The listing builds one solid part. Answer for the finished solid, in the listing's coordinates (mm). Face numbers are marked on the shaded views. A direction names the side the tool comes from. Give positions to 0.01 mm unless a question says otherwise; leave off trailing zeros. Write each loop counter-clockwise with the first axis right and the second up, starting at its lowest first coordinate (ties: lowest second). Pieces come first, ordered by that corner, then holes. Notation, with made-up numbers: (30.5, 51.25) -> (74.5, 51.25) arc R17 cw to (74.5, 81.25) -> close; hole circle Ø11 at (-5, 7). An arc over 180 degrees is marked (long way). Use CSV: the item, a comma, the result in double quotes. Start each with the question number.
from build123d import *

# Parameters (mm, degrees)
CLAMP_EXTRUDE_DEPTH     = 10
HOLE_R                  = 1.6
HOLES_CUT_EXTRUDE_DEPTH = 6
FILLET1_R               = 1


with BuildPart() as part:
    # Sketch4 → Clamp Extrude (new body)
    with BuildSketch(Plane(origin=(0, 0, 0), x_dir=(0, 0, -1), z_dir=(1, 0, 0))):
        with BuildLine():
            Line((-23.6125, 0), (-11.1125, 0))
            ThreePointArc((-11.1125, 0), (0, -11.1125), (11.1125, 0))
            Line((11.1125, 0), (23.6125, 0))
            Line((23.6125, 0), (23.6125, -5))
            Line((23.6125, -5), (13.789947652, -5))
            ThreePointArc((13.789947652, -5), (0, -14.668423782), (-13.789947652, -5))
            Line((-13.789947652, -5), (-23.6125, -5))
            Line((-23.6125, -5), (-23.6125, 0))
        make_face()
    extrude(amount=CLAMP_EXTRUDE_DEPTH)

    # Hole → Holes Cut-Extrude (cut, through all)
    with BuildSketch(Plane.XZ.offset(5)):
        with Locations((5, 18.701223826)):
            Circle(HOLE_R)
        with Locations((5, -18.701223826)):
            Circle(HOLE_R)
    extrude(amount=-HOLES_CUT_EXTRUDE_DEPTH, mode=Mode.SUBTRACT)

    # Fillet1
    fillet1_edges = [part.edges().sort_by_distance(p)[0] for p in [
        (0, -2.5, -23.6125),
        (0, -5, -18.701223826),
        (0, -14.668423782, 0),
        (10, -2.5, -23.6125),
        (5, -5, 13.789947652),
        (5, -5, 23.6125),
        (5, -5, -23.6125),
        (5, -5, -13.789947652),
        (10, -2.5, 23.6125),
        (10, -5, 18.701223826),
        (10, -14.668423782, 0),
        (0, -5, 18.701223826),
        (10, -5, -18.701223826),
        (0, -2.5, 23.6125),
    ]]
    fillet(fillet1_edges, radius=FILLET1_R)


solid = part.part
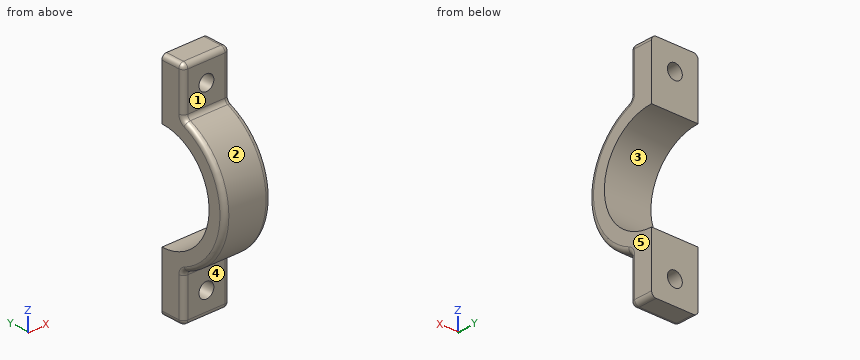
Q1. Section D-D on x = 1.5 is taken. Give the vertices of the cut face in (y, z) (1 decimal), then the cut area to 3 significant figures.
Q2. The mould has two halves that part along Z. Classify the marked faces 1, 2 and 3: +Z half, -Z half, draft (parallel to the pull), parting line (faces both ways), or undercut.
Q3. Straight lines are drawn through the part: L1, parallel to Z at x = 5, y = -2.6; L2, parallel to Z at x = 5, y = -3.2; L3, parallel to Y at x = 2.25, z = -18. For each, find the intervals that lie inside material, in ascending order.
Q4. Section B-B on y = -2.5 is taken. Give the vertices of the cut face in (x, z).
Q5. Section C-C on z = 0 is taken. Give the vertices of the cut face in (x, y), then the cut area to 3 significant figures.
Q6. For the marked faces 4 and 5, determine the directions among +Z, -Z, +X, -X, +Y, -Y from which every point of the face is accessible in a straight line to the end or side of a thin tool.
Q7. Flat-ended cylindrical pins translate along their axes: pin 1 Ø3 at (x, y) = (4.5, -9) entering from -Z; pin 2 Ø4 at (x, y) = (3.5, -12.5) entering from -Z; pin 3 Ø1.9 at (x, z) = (5, -18.7) entering from +Y; pin 4 Ø2.5 at (x, z) = (5.5, -17) entering from -Y. Find the tip coordinate at first contact, or state that the pin passes through.
Q8. Section A-A on x = 5 is taken. Give the vertices of the cut face in (y, z) (1 decimal).
Output:
1,outline,"(-5.6, -13.6) arc R1 cw to (-5, -14.5) -> (-5, -22.6) arc R1 ccw to (-4, -23.6) -> (0, -23.6) -> (0, -11.1) arc R11.1 cw to (0, 11.1) -> (0, 23.6) -> (-4, 23.6) arc R1 ccw to (-5, 22.6) -> (-5, 14.5) arc R1 cw to (-5.6, 13.6) arc R14.7 ccw to start"
1,area,"236 mm²"
2,face 1,"draft"
2,face 2,"parting line"
2,face 3,"undercut"
3,L1,"-23.61 to -20.3, -17.1 to -10.8, 10.8 to 17.1, 20.3 to 23.61"
3,L2,"-23.61 to -20.3, -17.1 to -10.64, 10.64 to 17.1, 20.3 to 23.61"
3,L3,"-5 to 0"
4,outline,"(0, -22.61) arc R1 ccw to (1, -23.61) -> (9, -23.61) arc R1 ccw to (10, -22.61) -> (10, -10.83) -> (0, -10.83) -> close; (0, 10.83) -> (10, 10.83) -> (10, 22.61) arc R1 ccw to (9, 23.61) -> (1, 23.61) arc R1 ccw to (0, 22.61) -> close; hole circle Ø3.2 at (5, -18.7); hole circle Ø3.2 at (5, 18.7)"
5,outline,"(0, -13.67) arc R1 ccw to (1, -14.67) -> (9, -14.67) arc R1 ccw to (10, -13.67) -> (10, -11.11) -> (0, -11.11) -> close"
5,area,"35.1 mm²"
6,face 4,"-Z, +X, -X, -Y"
6,face 5,"+Z, -Z, +X, +Y, -Y"
7,pin 1,"z = -12.61"
7,pin 2,"z = -10.24"
7,pin 3,"through"
7,pin 4,"y = -5"
8,outline,"(-5.6, -13.6) arc R1 cw to (-5, -14.5) -> (-5, -17.1) -> (0, -17.1) -> (0, -11.1) arc R11.1 cw to (0, 11.1) -> (0, 17.1) -> (-5, 17.1) -> (-5, 14.5) arc R1 cw to (-5.6, 13.6) arc R14.7 ccw to start; (-5, -22.6) arc R1 ccw to (-4, -23.6) -> (0, -23.6) -> (0, -20.3) -> (-5, -20.3) -> close; (-5, 20.3) -> (0, 20.3) -> (0, 23.6) -> (-4, 23.6) arc R1 ccw to (-5, 22.6) -> close"
